Could you check a few things on this model? Use its own coordinates, in mm. A direction names the side the tool comes from. Round coordinates to 2 decimals unless told otherwise and drop trailing zeros. Write each loop counter-clockwise with the first axis right and the second up, starting at its lowest first coordinate (ties: lowest second). Pieces come first, ordered by that corner, then holes. Notation, with made-up numbers: M 46,-6 L 96,-6 A26 ccw 96,17 Z; hole C 79.5,21 d1. An arc over 180 degrees is marked long. One line per item, written item: value. Start each with the question number.
(1) I want a section at C-C on z = 14. Please give me the cut outline in (x, y), and give its area (3 significant figures).
(2) I want a section at D-D on y = 77.5. Please give me the cut outline in (x, z).
(3) I want a section at B-B on y = 39.5. Please give me the cut outline in (x, z), and give its area (3 significant figures).
(4) If I drill on L1, parallel to Y at x = 12.5, z = 2.95; L2, parallel to X at y = 36.2, z = 4.4; L3, parallel to X at y = 17, z = 3.5, over which ranges is the centre line in solid material (lowest first)?
(5) Which directions (+Z, -Z, +X, -X, +Y, -Y) give clear straight access to the entire face, cutting with the end or side of a thin tool? Please do faces 4 (the face through (11, 115.04, 5)), 5 (the face through (0, 75, 3)), 6 (the face through (23.406, 16, 2)), 7 (the face through (7, 20, 1)), 8 (the face through (12, 48, 5)).
(6) Thinking about a two-plate mould opening in X: for faces 1 (the face through (13, 22, 4)), 2 (the face through (2, 1, 3)), 3 (the face through (13, 116, 20)), which applies, released by +X, released by -X, zero draft, split by the parting line, or undercut?
(7) I'm going to push flat-ended pins straight in: pin 1 Ø9 at (x, y) = (17, 22.5) entering from -Z; pin 2 Ø1 at (x, z) = (19, 14) entering from +Y; pin 3 Ø1.5 at (x, y) = (7, 102.5) entering from +Z; pin 4 Ø0.5 at (x, y) = (12.5, 36) entering from +Z. Where does each tip first touch, or does it pass through?
(8) I want a section at A-A on y = 15. Please give me the cut outline in (x, z).
```python
from build123d import *

# Parameters (mm, degrees)
SKICA1_W                 = 25
SKICA1_H                 = 120
P_IDAT_VYSUNUT_M1_DEPTH  = 5
SKICA2_W                 = 25
SKICA2_H                 = 15
P_IDAT_VYSUNUT_M2_DEPTH  = 20
ZAOBLIT5_R               = 5
ZAOBLIT6_R               = 5
ODEBRAT_VYSUNUT_M2_DEPTH = 20
ZAOBLIT7_R               = 10
ZAOBLIT8_R               = 10
SKICA4_W                 = 3
SKICA4_H                 = 10
ODEBRAT_VYSUNUT_M3_DEPTH = 3
ODEBRAT_VYSUNUT_M4_DEPTH = 2
ODEBRAT_START            = -3
SKICA7_R                 = 0.5
ODEBRAT_VYSUNUT_M5_DEPTH = 2.8
SKICA8_R                 = 3.75
ODEBRAT_VYSUNUT_M6_DEPTH = 2
SKICA9_W                 = 7.5
SKICA9_H                 = 8
ODEBRAT_VYSUNUT_M7_DEPTH = 125.197423617


with BuildPart() as part:
    # Skica1 → Přidat vysunutím1 (new body)
    with BuildSketch(Plane.XY):
        with Locations((12.5, 60)):
            Rectangle(SKICA1_W, SKICA1_H)
    extrude(amount=P_IDAT_VYSUNUT_M1_DEPTH)

    # Skica2 → Přidat vysunutím2 (add)
    with BuildSketch(Plane(origin=(0, 0, 0), x_dir=(-1, 0, 0), z_dir=(0, 0, -1))):
        with Locations((-12.5, 112.5)):
            Rectangle(SKICA2_W, SKICA2_H)
    extrude(amount=-P_IDAT_VYSUNUT_M2_DEPTH)

    # Zaoblit5
    zaoblit5_edges = [part.edges().sort_by_distance(p)[0] for p in [
        (25, 0, 2.5),
    ]]
    fillet(zaoblit5_edges, radius=ZAOBLIT5_R)

    # Zaoblit6
    zaoblit6_edges = [part.edges().sort_by_distance(p)[0] for p in [
        (0, 0, 2.5),
    ]]
    fillet(zaoblit6_edges, radius=ZAOBLIT6_R)

    # Skica3 → Odebrat vysunutím2 (cut)
    with BuildSketch(Plane.XY.offset(20)):
        with BuildLine():
            Line((1.5, 118.04), (23.5, 118.04))
            ThreePointArc((23.5, 118.04), (24.1, 118.64), (23.5, 119.24))
            ThreePointArc((23.5, 119.24), (23.12, 119.62), (23.5, 120))
            Line((23.5, 120), (1.5, 120))
            ThreePointArc((1.5, 120), (1.88, 119.62), (1.5, 119.24))
            ThreePointArc((1.5, 119.24), (0.9, 118.64), (1.5, 118.04))
        make_face()
    extrude(amount=-ODEBRAT_VYSUNUT_M2_DEPTH, mode=Mode.SUBTRACT)

    # Zaoblit7
    zaoblit7_edges = [part.edges().sort_by_distance(p)[0] for p in [
        (12.5, 105, 20),
    ]]
    fillet(zaoblit7_edges, radius=ZAOBLIT7_R)

    # Zaoblit8
    zaoblit8_edges = [part.edges().sort_by_distance(p)[0] for p in [
        (12.5, 105, 5),
    ]]
    fillet(zaoblit8_edges, radius=ZAOBLIT8_R)

    # Skica4 → Odebrat vysunutím3 (cut)
    with BuildSketch(Plane(origin=(0, 118.04, 0), x_dir=(1, 0, 0), z_dir=(0, 1, 0))):
        with Locations((10.62, -5)):
            Rectangle(SKICA4_W, SKICA4_H)
    extrude(amount=-ODEBRAT_VYSUNUT_M3_DEPTH, mode=Mode.SUBTRACT)

    # Skica5 → Odebrat vysunutím4 (cut)
    with BuildSketch(Plane.XY):
        Polygon((11, 43), (9.272727273, 24), (15.727272727, 24), (14, 43), align=None)
        with BuildLine():
            Line((5.5, 24), (5.5, 20))
            ThreePointArc((5.5, 20), (3.5, 22), (5.5, 24))
        make_face()
        Polygon((9.09375, 20), (9, 21), (9.272727273, 24), (5.5, 24), (5.5, 20), align=None)
        Polygon((9.272727273, 24), (9, 21), (16, 21), (15.727272727, 24), align=None)
        Polygon((16, 21), (9, 21), (9.09375, 20), (15.90625, 20), align=None)
        Polygon((15.727272727, 24), (16, 21), (15.90625, 20), (19.5, 20), (19.5, 24), align=None)
        with BuildLine():
            ThreePointArc((19.5, 24), (21.5, 22), (19.5, 20))
            Line((19.5, 20), (19.5, 24))
        make_face()
        Polygon((15.90625, 20), (9.09375, 20), (10.5, 5), (14.5, 5), align=None)
    extrude(amount=ODEBRAT_VYSUNUT_M4_DEPTH, mode=Mode.SUBTRACT)

    # Skica7 → Odebrat vysunutím5 (cut)
    with BuildSketch(Plane(origin=(0, 0, 2), x_dir=(-1, 0, 0), z_dir=(0, 0, -1)).offset(ODEBRAT_START)):
        with Locations(Location((-12.5, 36.2, 0), (0, 0, 180))):
            Circle(SKICA7_R)
        with Locations(Location((-12.5, 9.7, 0), (0, 0, 180))):
            Circle(SKICA7_R)
    extrude(amount=ODEBRAT_VYSUNUT_M5_DEPTH, mode=Mode.SUBTRACT)

    # Skica8 → Odebrat vysunutím6 (cut)
    with BuildSketch(Plane(origin=(0, 0, 2), x_dir=(-1, 0, 0), z_dir=(0, 0, -1))):
        with Locations((-12.5, 22)):
            Circle(SKICA8_R)
    extrude(amount=-ODEBRAT_VYSUNUT_M6_DEPTH, mode=Mode.SUBTRACT)

    # Skica9 → Odebrat vysunutím7 (cut, through all)
    with BuildSketch(Plane(origin=(0, 0, 0), x_dir=(-1, 0, 0), z_dir=(0, 0, -1))):
        with Locations((-19.65625, 16)):
            Rectangle(SKICA9_W, SKICA9_H)
    extrude(amount=-ODEBRAT_VYSUNUT_M7_DEPTH, mode=Mode.SUBTRACT)


solid = part.part
```
Found:
1. outline: M 0,105.83 L 25,105.83 L 25,120 L 23.5,120 A0.38 ccw 23.5,119.24 A0.6 cw 23.5,118.04 L 1.5,118.04 A0.6 cw 1.5,119.24 A0.38 ccw 1.5,120 L 0,120 Z
1. area: 310 mm²
2. outline: M 0,0 L 25,0 L 25,5 L 0,5 Z
3. outline: M 0,0 L 10.68,0 L 10.68,2 L 14.32,2 L 14.32,0 L 25,0 L 25,5 L 0,5 Z
3. area: 118 mm²
4. L1: y = 0 to 9.2, 10.2 to 18.25, 25.75 to 35.7, 36.7 to 118.04
4. L2: x = 0 to 12, 13 to 25
4. L3: x = 0 to 15.91, 23.41 to 25
5. face 4: -Z, +Y
5. face 5: +Z, -Z, -X, +Y, -Y
5. face 6: +Z, -Z
5. face 7: -Z
5. face 8: +Z, +X, -X, -Y
6. face 1: undercut
6. face 2: released by -X
6. face 3: zero draft
7. pin 1: stops at z = 0
7. pin 2: stops at y = 118.04
7. pin 3: stops at z = 8.52
7. pin 4: stops at z = 2.2
8. outline: M 0,0 L 9.56,0 L 9.56,2 L 15.44,2 L 15.44,0 L 15.91,0 L 15.91,5 L 0,5 Z; M 23.41,0 L 25,0 L 25,5 L 23.41,5 Z
